Here's how the part is built. I have some questions about the finished solid (model axes, mm). A direction names the side the tool comes from. Round coordinates to 2 decimals unless told otherwise and drop trailing zeros. Write each loop counter-clockwise with the first axis right and the second up, starting at its lowest first coordinate (ties: lowest second). Pieces come first, ordered by that corner, then holes. Notation, with made-up numbers: (38.5, 58) -> (56.5, 58) arc R15 cw to (56.5, 70) -> close; hole circle Ø5 at (-39, 42.5). An arc over 180 degrees is marked (long way). Answer as CSV lines item,"result".
from build123d import *

# Parameters (mm, degrees)
SKETCH1_W           = 10
SKETCH1_H           = 10
REVOLVE1_ANGLE      = 180
BOSS_EXTRUDE1_START = 10
SKETCH3_R           = 7
SKETCH3_R_2         = 0.094269149
BOSS_EXTRUDE1_DEPTH = 60
SKETCH5_R           = 2.1
CUT_EXTRUDE1_DEPTH  = 6
SKETCH6_R           = 2.1
CUT_EXTRUDE2_DEPTH  = 6
BOSS_EXTRUDE3_DEPTH = 2
SKETCH14_R          = 1.6
CUT_EXTRUDE5_DEPTH  = 2


with BuildPart() as part:
    # Sketch1 → Revolve1 (revolve)
    with BuildSketch(Plane(origin=(0, 0, 0), x_dir=(1, 0, 0), z_dir=(0, 1, 0))):
        with Locations((-9.8, 5)):
            Rectangle(SKETCH1_W, SKETCH1_H)
    revolve(axis=Axis((0, 0, 3.39750235), (0, 0, -1)), revolution_arc=REVOLVE1_ANGLE)

    # Sketch3 → Boss-Extrude1 (add)
    with BuildSketch(Plane(origin=(0, 0, 0), x_dir=(1, 0, 0), z_dir=(0, 1, 0)).offset(BOSS_EXTRUDE1_START)):
        with Locations((0, 5)):
            Circle(SKETCH3_R)
        with Locations((0, 5)):
            Circle(SKETCH3_R_2, mode=Mode.SUBTRACT)
    extrude(amount=BOSS_EXTRUDE1_DEPTH)

    # Sketch5 → Cut-Extrude1 (cut)
    with BuildSketch(Plane.XZ):
        with Locations((9.8, -5)):
            Circle(SKETCH5_R)
    extrude(amount=-CUT_EXTRUDE1_DEPTH, mode=Mode.SUBTRACT)

    # Sketch6 → Cut-Extrude2 (cut)
    with BuildSketch(Plane.XZ):
        with Locations((-9.8, -5)):
            Circle(SKETCH6_R)
    extrude(amount=-CUT_EXTRUDE2_DEPTH, mode=Mode.SUBTRACT)

    # Sketch11 → Boss-Extrude3 (add)
    with BuildSketch(Plane(origin=(0, 70, 0), x_dir=(1, 0, 0), z_dir=(0, 1, 0))):
        with BuildLine():
            Line((-15.699935159, 20), (15.51139686, 20))
            ThreePointArc((15.51139686, 20), (30.51139686, 5), (15.51139686, -10))
            Line((15.51139686, -10), (-15.699935159, -10))
            ThreePointArc((-15.699935159, -10), (-30.699935159, 5), (-15.699935159, 20))
        make_face()
    extrude(amount=BOSS_EXTRUDE3_DEPTH)

    # Sketch14 → Cut-Extrude5 (cut)
    with BuildSketch(Plane(origin=(0, 72, 0), x_dir=(1, 0, 0), z_dir=(0, 1, 0))):
        with Locations((-15.699935159, 5)):
            Circle(SKETCH14_R)
        with Locations((15.51139686, 5)):
            Circle(SKETCH14_R)
    extrude(amount=-CUT_EXTRUDE5_DEPTH, mode=Mode.SUBTRACT)


solid = part.part
Item 1: Suppose I cut it at B-B, the plane z = -1.5. List the corners of the cut face in (x, y) for me, then the cut area to 3 significant figures.
Results found:
outline,"(-30.29, 70) -> (-6.06, 70) -> (-6.06, 13.5) arc R14.8 ccw to (-14.8, 0) -> (-4.8, 0) arc R4.8 cw to (4.8, 0) -> (14.8, 0) arc R14.8 ccw to (6.06, 13.5) -> (6.06, 70) -> (30.1, 70) -> (30.1, 72) -> (-30.29, 72) -> close"
area,"1,100 mm²"
Item 2: Will these pins go through, and if not, where does the flat tip stop? pin 1 (2 mm diameter, centred on y = 36, z = -10, fed in from -X); pin 2 (3 mm diameter, centred on x = -24, z = -4.5, fed in from -Y); pin 3 (2 mm diameter, centred on x = -1, z = 0.5, fed in from -Y); pin 4 (4.5 mm diameter, centred on x = -9, z = -4.5, fed in from -Y).
Results found:
pin 1,"stops at x = -5.74"
pin 2,"stops at y = 70"
pin 3,"stops at y = 4.42"
pin 4,"stops at y = 0"
Item 3: If we mould it in two halves opening along Y, with no side actions, what happens to faces 4 (the cylindrical face through (-12.147, 8.455, -5.07)), 5 (the cylindrical face through (-0.1, 4.8, -5.1)), 6 (the flat face through (0, 6, 0)), 7 (the cylindrical face through (6.677, 39.58, -7.103))? For each: pulls with the +Y half, pulls with the -Y half, needs draft (parallel to the pull), parting line crosses it, or undercut.
Results found:
face 4,"undercut"
face 5,"pulls with the -Y half"
face 6,"needs draft"
face 7,"undercut"
Item 4: For faces 1 (the flat face through (0, 10, -11)), 2 (the cylindrical face through (-8.831, 2.958, -6.863)), 3 (the flat face through (0, 10, 1)), which set-ups out of +Z, -Z, +X, -X, +Y, -Y let a thin tool reach every point of the face, with its end or its side?
Results found:
face 1,"-Z, +X, -X, -Y"
face 2,"-Y"
face 3,"+Z, +X, -X, -Y"
Item 5: Suppose I cut it at A-A, the plane x = 9.8. List the corners of the cut face in (y, z) for me.
Results found:
outline,"(0, -10) -> (11.09, -10) -> (11.09, 0) -> (0, 0) -> (0, -2.9) -> (6, -2.9) -> (6, -7.1) -> (0, -7.1) -> close; (70, -20) -> (72, -20) -> (72, 10) -> (70, 10) -> close"
Item 6: Suppose I cut it at D-D, the plane x = -8.5. List the corners of the cut face in (y, z) for me, then the cut area to 3 significant figures.
Results found:
outline,"(0, -10) -> (12.12, -10) -> (12.12, 0) -> (0, 0) -> (0, -3.35) -> (6, -3.35) -> (6, -6.65) -> (0, -6.65) -> close; (70, -20) -> (72, -20) -> (72, 10) -> (70, 10) -> close"
area,"161 mm²"
Item 7: Suppose I cut it at C-C, the plane y = 30. List the corners of the cut face in (x, z) for me.
Results found:
outline,"circle Ø14 at (0, -5); hole circle Ø0.19 at (0, -5)"
Item 8: I need wall thicknesses on L1, parallel to X at y = 71.25, z = -5; L2, parallel to Z at x = 9.8, y = 4.5; L3, parallel to Y at x = -16.5, z = -13. Which ranges of each line are inside material? Lowest first, please.
Results found:
L1,"x = -30.7 to -17.3, -14.1 to 13.91, 17.11 to 30.51"
L2,"z = -10 to -7.1, -2.9 to 0"
L3,"y = 70 to 72"
